Build history of the part. All positions in model axes, mm. Round coordinates to 2 decimals unless told otherwise and drop trailing zeros. Write each loop counter-clockwise with the first axis right and the second up, starting at its lowest first coordinate (ties: lowest second). Pieces come first, ordered by that corner, then holes. Notation, with made-up numbers: (48, 79) -> (84, 79) arc R14 cw to (84, 90) -> close; hole circle Ø10 at (61.25, 20). An arc over 180 degrees is marked (long way). Answer in a Markdown table with one row per item.
```python
from build123d import *

# Parameters (mm, degrees)
BOX_W              = 500
BOX_H              = 240
BOX_DEPTH          = 14.7
POCKET_DEPTH       = 14.701
SKETCH001_R        = 5
POCKET001_DEPTH    = 6
SKETCH001001_R     = 3.25
POCKET002_DEPTH    = 14.701
POCKET003001_DEPTH = 5


with BuildPart() as part:
    # Box → Box (new body)
    with BuildSketch(Plane.XY):
        with Locations((250, 120)):
            Rectangle(BOX_W, BOX_H)
    extrude(amount=BOX_DEPTH)

    # Sketch → Pocket (cut, through all)
    with BuildSketch(Plane.XY.offset(14.7)):
        with BuildLine():
            Line((10.001, 0), (10.001, 19.857041))
            ThreePointArc((10.001, 19.857041), (5.607587, 30.463616), (-4.999, 34.857))
            Line((-4.999, 0), (-4.999, 34.857))
            Line((10.001, 0), (-4.999, 0))
        make_face()
    extrude(amount=-POCKET_DEPTH, mode=Mode.SUBTRACT)

    # Sketch001 → Pocket001 (cut)
    with BuildSketch(Plane.XY.offset(14.7)):
        with Locations((17, 225)):
            Circle(SKETCH001_R)
        with Locations((17, 85)):
            Circle(SKETCH001_R)
        with Locations((17, 15)):
            Circle(SKETCH001_R)
        with Locations((17, 155)):
            Circle(SKETCH001_R)
        with Locations((493, 155)):
            Circle(SKETCH001_R)
        with Locations((493, 85)):
            Circle(SKETCH001_R)
        with Locations((493, 225)):
            Circle(SKETCH001_R)
        with Locations((493, 15)):
            Circle(SKETCH001_R)
    extrude(amount=-POCKET001_DEPTH, mode=Mode.SUBTRACT)

    # Sketch001001 → Pocket002 (cut, through all)
    with BuildSketch(Plane.XY.offset(14.7)):
        with Locations((17, 225)):
            Circle(SKETCH001001_R)
        with Locations((17, 85)):
            Circle(SKETCH001001_R)
        with Locations((17, 15)):
            Circle(SKETCH001001_R)
        with Locations((17, 155)):
            Circle(SKETCH001001_R)
        with Locations((493, 155)):
            Circle(SKETCH001001_R)
        with Locations((493, 85)):
            Circle(SKETCH001001_R)
        with Locations((493, 225)):
            Circle(SKETCH001001_R)
        with Locations((493, 15)):
            Circle(SKETCH001001_R)
    extrude(amount=-POCKET002_DEPTH, mode=Mode.SUBTRACT)

    # Sketch001002 → Pocket003001 (cut)
    with BuildSketch(Plane.XY.offset(14.7)):
        with BuildLine():
            Line((395, 125), (0, 125))
            Line((0, 125), (0, 115))
            Line((0, 115), (395, 115))
            ThreePointArc((395, 115), (400.000017, 120), (395, 125))
        make_face()
    extrude(amount=-POCKET003001_DEPTH, mode=Mode.SUBTRACT)


solid = part.part
```
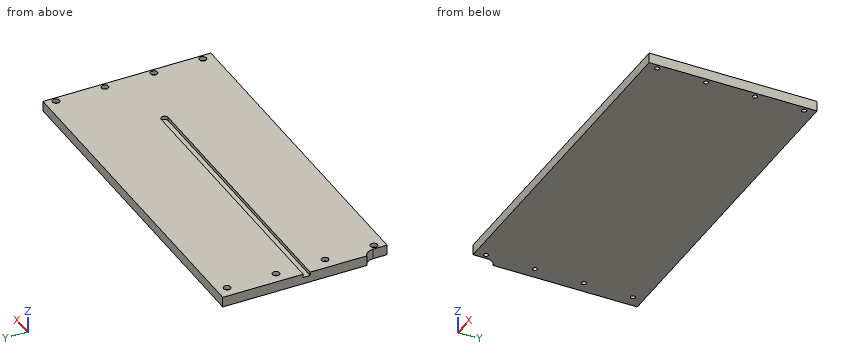
Q1. Saw through at A-A on y = 120. Write the cut outline in (x, z), plus the area to 3 significant figures.
A:
| item | result |
|---|---|
| outline | (0, 0) -> (500, 0) -> (500, 14.7) -> (400, 14.7) -> (400, 9.7) -> (0, 9.7) -> close |
| area | 5,350 mm² |
Q2. Saw through at B-B on y = 27.5. Write the cut outline in (x, z), plus the area to 3 significant figures.
A:
| item | result |
|---|---|
| outline | (7.91, 0) -> (500, 0) -> (500, 14.7) -> (7.91, 14.7) -> close |
| area | 7,230 mm² |
Q3. Wall check: line 1 (Y direction, x = 17, z = 5.5); line 2 (Y direction, x = 493, z = 11.45); line 3 (X direction, y = 155, z = 3). Give the ranges that are in metal, low to high. Write a range as [from, to].
A:
| item | result |
|---|---|
| line 1 | [0, 11.75], [18.25, 81.75], [88.25, 151.75], [158.25, 221.75], [228.25, 240] |
| line 2 | [0, 10], [20, 80], [90, 150], [160, 220], [230, 240] |
| line 3 | [0, 13.75], [20.25, 489.75], [496.25, 500] |
Q4. Drop flat-ended pins along their axis: P1, Ø4, axis at x = 493, y = 15, coming from the +Z side; P2, Ø9, axis at x = 17, y = 225, coming from the +Z side. Give the stop position or say it passes through.
A:
| item | result |
|---|---|
| P1 | through |
| P2 | z = 8.7 |
